```python
from build123d import *

# Parameters (mm, degrees)
F0_W          = 36.3989807665
F0_H          = 46.9546951354
F1_ANGLE_BACK = 150
F1_ANGLE      = 300
F2_R          = 6.3818530104
F3_DEPTH      = 25.4


with BuildPart() as f1:
    # F0 (on Front) → F1 (revolve)
    with BuildSketch(Plane.XZ, mode=Mode.PRIVATE) as f1_sk:
        with Locations((18.1994903833, 0)):
            Rectangle(F0_W, F0_H)
    revolve(f1_sk.sketch.rotate(Axis((0, 0, 0), (0, 0, -1)), -F1_ANGLE_BACK), axis=Axis((0, 0, 0), (0, 0, -1)), revolution_arc=F1_ANGLE)

    # F2 (on Top) → F3 (join, symmetric)
    with BuildSketch(Plane.XY):
        with Locations((-6.0975761153, 26.0735042393)):
            Circle(F2_R)
    extrude(amount=F3_DEPTH, both=True)


solid = f1.part
```
Check sheet for the modelled part. Datum: model origin and axes. Units: mm. A direction names the side the tool comes from. Give positions to 0.01 mm unless a question says otherwise; leave off trailing zeros. Write each loop counter-clockwise with the first axis right and the second up, starting at its lowest first coordinate (ties: lowest second). Pieces come first, ordered by that corner, then holes.
Item 1: Access from +Z, -Z, +X, -X, +Y, -Y to the whole of each face (thin tool, end or side, straight path). Record for faces 1 (the face through (-6.93, 32.4, 24.45)), 2 (the face through (-6.93, 32.4, -24.43)), 3 (the face through (-6, 26, 25.4)), 4 (the face through (-15.54, 8.97, 0.33)).
Item 2: Gauge pin test, flat ends, axial feed: pin 1 (4 mm diameter, centred on x = -2.5, y = 15, fed in from +Z); pin 2 (1.5 mm diameter, centred on x = -4, z = 6.5, fed in from -Y); pin 3 (1 mm diameter, centred on x = 2, z = 17.5, fed in from -Y). Record the tip position at first contact, or that the pin passes through.
Item 3: Cross-section at A-A (x = -17). Enter the section's corners in (y, z).
Item 4: Scan lines: L1, parallel to Z at x = 20, y = 0.5; L2, parallel to Y at x = -25, z = 7.5; L3, parallel to Y at x = -24, z = 16. Record each from-to range of solid material in increasing order.
Item 5: Cross-section at C-C (x = -25.5). Enter the section's corners in (y, z).
Item 6: Draft check along Y on faces 5 (the face through (36.375, 1.334, 0.329)), 6 (the face through (-15.54, -8.97, 0.33)), 7 (the face through (-6, 26, -25.4)). Enter one of: released by +Y, released by -Y, zero draft, split by the parting line, or undercut.
Item 7: Cross-section at D-D (y = -10). Enter the section's corners in (x, z).
Item 8: Cross-section at B-B (z = -16). Enter the section's corners in (x, y), and give its area (3 significant figures).
Report:
1. face 1: +Z
1. face 2: -Z
1. face 3: +Z, +X, -X, +Y, -Y
1. face 4: +Z, -Z, -X
2. pin 1: stops at z = 23.48
2. pin 2: stops at y = -36.25
2. pin 3: stops at y = -36.37
3. outline: (-32.19, -23.48) - (-9.81, -23.48) - (-9.81, 23.48) - (-32.19, 23.48) - close; (9.81, -23.48) - (32.19, -23.48) - (32.19, 23.48) - (9.81, 23.48) - close
4. L1: z = -23.48 to 23.48
4. L2: y = -26.46 to -14.43, 14.43 to 26.46
4. L3: y = -27.37 to -13.86, 13.86 to 27.37
5. outline: (-25.97, -23.48) - (-14.72, -23.48) - (-14.72, 23.48) - (-25.97, 23.48) - close; (14.72, -23.48) - (25.97, -23.48) - (25.97, 23.48) - (14.72, 23.48) - close
6. face 5: split by the parting line
6. face 6: undercut
6. face 7: zero draft
7. outline: (-17.32, -23.48) - (35, -23.48) - (35, 23.48) - (-17.32, 23.48) - close
8. outline: (-31.52, -18.2) arc R36.4 ccw (long way) to (-31.52, 18.2) - (0, 0) - close
8. area: 3,470 mm2
